Could you check a few things on this drawing? It's one solid part, dimensions in mm from its lowest x, y, z. A direction names the side the tool comes from. Give positions to 0.01 mm unless a question says otherwise; leave off trailing zeros. Order: outer loops, then holes, each group sorted by start corner. A loop starts at its lowest first (then second) coordinate and runs counter-clockwise, first axis right, second up.
Item 1: If we mould it in two halves opening along X, with no side actions, what happens to the marked faces 1, 2, 3 and 4? For each: +X half, -X half, draft (parallel to the pull), parting line (faces both ways), or undercut.
Item 2: I want a section at B-B, the plane z = 1. Write out the boundary of the cut face in (x, y), then the cut area to 3 significant figures.
Item 3: Which directions (+Z, -Z, +X, -X, +Y, -Y) give clear straight access to the entire face, cutting with the end or side of a thin tool? Please do the marked faces 5, 6, 7, 8 and 9.
Item 4: I want a section at D-D, the plane y = 27. Write out the boundary of the cut face in (x, z).
Item 5: I want a section at C-C, the plane z = 5.25. Write out the boundary of the cut face in (x, y), then the cut area to 3 significant figures.
Item 6: If I drill on line 1 along Y through (x, z) = (63.5, 11.2); line 2 along X through (y, z) = (22.5, 3.5); line 3 along X through (y, z) = (14.5, 2.25), over which ranges is the centre line in solid material (lowest first)?
Item 7: I want a section at A-A, the plane x = 63.5. Write out the boundary of the cut face in (y, z).
Item 8: I'm going to push flat-ended pins straight in: pin 1 Ø2 at (y, z) = (31, 7.5) entering from -X; pin 2 Ø4 at (y, z) = (21, 5) entering from +X; pin 3 Ø3 at (y, z) = (27.5, 5.5) entering from +X; pin 4 Ø3.5 at (x, y) = (63.5, 33.5) entering from +Z. Where does each tip first touch, or does it pass through?
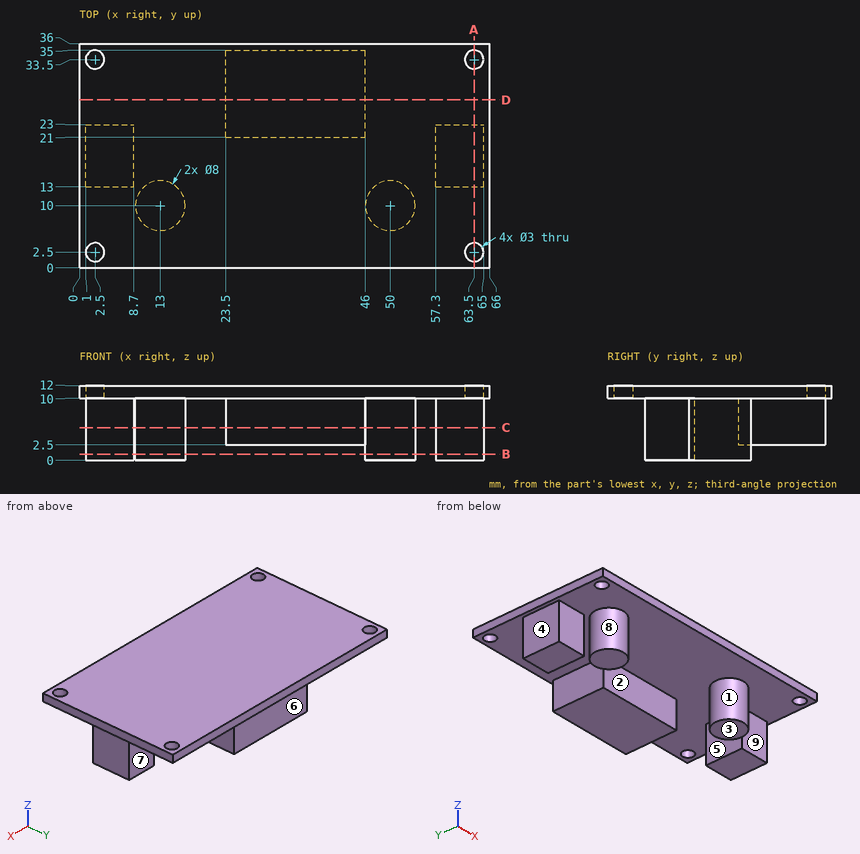
Results list:
1. face 1: undercut
1. face 2: undercut
1. face 3: draft
1. face 4: -X half
2. outline: (1, 13) - (8.7, 13) - (8.7, 23) - (1, 23) - close; circle Ø8 at (13, 10); circle Ø8 at (50, 10); (57.3, 13) - (65, 13) - (65, 23) - (57.3, 23) - close
2. area: 255 mm2
3. face 5: -Z, +Y, -Y
3. face 6: -Z, +X, -X, +Y
3. face 7: -Z, +X, +Y
3. face 8: -Z
3. face 9: -Z, +X, -Y
4. outline: (0, 10) - (23.5, 10) - (23.5, 2.5) - (46, 2.5) - (46, 10) - (66, 10) - (66, 12) - (0, 12) - close
5. outline: (1, 13) - (8.7, 13) - (8.7, 23) - (1, 23) - close; circle Ø8 at (13, 10); (23.5, 21) - (46, 21) - (46, 35) - (23.5, 35) - close; circle Ø8 at (50, 10); (57.3, 13) - (65, 13) - (65, 23) - (57.3, 23) - close
5. area: 570 mm2
6. line 1: y = 0 to 1, 4 to 32, 35 to 36
6. line 2: x = 1 to 8.7, 23.5 to 46, 57.3 to 65
6. line 3: x = 1 to 8.7, 57.3 to 65
7. outline: (0, 10) - (1, 10) - (1, 12) - (0, 12) - close; (4, 10) - (13, 10) - (13, 0) - (23, 0) - (23, 10) - (32, 10) - (32, 12) - (4, 12) - close; (35, 10) - (36, 10) - (36, 12) - (35, 12) - close
8. pin 1: stops at x = 23.5
8. pin 2: stops at x = 65
8. pin 3: stops at x = 46
8. pin 4: stops at z = 12
